CAD build for the part. Positions are in the model's coordinates, mm. Face numbers are marked on the shaded views. A direction names the side the tool comes from. Round coordinates to 2 decimals unless told otherwise and drop trailing zeros. Loops run counter-clockwise (first coordinate to the right, second up) from the corner with the lowest first, then second, coordinate; pieces in that order, holes last. Notation, with made-up numbers: M 60,-20.75 L 92,-20.75 A16 ccw 92,-11.75 Z; hole C 52,-20.5 d5. An arc over 180 degrees is marked long. One line per item, written item: value. Start each with the question number.
from build123d import *

# Parameters (mm, degrees)
SKETCH1_W                      = 59.28
SKETCH1_H                      = 38.1
BOSS_EXTRUDE2_DEPTH            = 29.26
SKETCH2_W                      = 15
SKETCH2_H                      = 38.1
BOSS_EXTRUDE3_DEPTH            = 4
SKETCH4_W                      = 44.28
SKETCH4_H                      = 25.7
CUT_EXTRUDE7_DEPTH             = 27.26
SKETCH7_R                      = 4.75
SKETCH8_R                      = 4.807692308
BOSS_EXTRUDE4_DEPTH            = 2
BOSS_EXTRUDE5_DEPTH            = 2
SKETCH15_W                     = 44.28
SKETCH15_H                     = 2
CUT_EXTRUDE9_DEPTH             = 2
BOSS_EXTRUDE6_DEPTH            = 1
F_2_0MM_DOWEL_HOLE1_AT_2_COUNT = 2
F_2_0MM_DOWEL_HOLE1_AT_2_PITCH = 20.32
LPATTERN1_COUNT                = 2
LPATTERN1_PITCH                = 33.15
SKETCH20_W                     = 25.7
SKETCH20_H                     = 27.26
SKETCH20_W_2                   = 14
SKETCH20_H_2                   = 14
CUT_EXTRUDE10_DEPTH            = 11


with BuildPart() as part:
    # Sketch1 → Boss-Extrude2 (new body)
    with BuildSketch(Plane(origin=(0, 0, 0), x_dir=(1, 0, 0), z_dir=(0, 1, 0))):
        with Locations((29.64, 19.05)):
            Rectangle(SKETCH1_W, SKETCH1_H)
    extrude(amount=BOSS_EXTRUDE2_DEPTH)

    # Sketch2 → Boss-Extrude3 (add)
    with BuildSketch(Plane(origin=(0, 29.26, 0), x_dir=(1, 0, 0), z_dir=(0, 1, 0))):
        with Locations((51.78, 19.05)):
            Rectangle(SKETCH2_W, SKETCH2_H)
    extrude(amount=BOSS_EXTRUDE3_DEPTH)

    # Sketch4 → Cut-Extrude7 (cut)
    with BuildSketch(Plane(origin=(0, 29.26, 0), x_dir=(1, 0, 0), z_dir=(0, 1, 0))):
        with Locations((22.14, 19.05)):
            Rectangle(SKETCH4_W, SKETCH4_H)
    extrude(amount=-CUT_EXTRUDE7_DEPTH, mode=Mode.SUBTRACT)

    # Sketch7 → Cut-Loft2 section 0
    with BuildSketch(Plane(origin=(59.28, 0, 0), x_dir=(0, 0, -1), z_dir=(1, 0, 0))):
        with Locations((19.05, 16.63)):
            Circle(SKETCH7_R)
    # Sketch8 → Cut-Loft2 section 1
    with BuildSketch(Plane.ZY.offset(-44.28)):
        with Locations((-19.05, 16.556791368)):
            Circle(SKETCH8_R)
    loft(mode=Mode.SUBTRACT)

    # Sketch13 → Boss-Extrude4 (add)
    with BuildSketch(Plane.XY):
        Polygon((0, 29.26), (0, 0), (59.28, 0), (59.28, 29.26), (59.28, 33.26), (0, 33.26), align=None)
    extrude(amount=BOSS_EXTRUDE4_DEPTH)

    # Sketch14 → Boss-Extrude5 (add)
    with BuildSketch(Plane(origin=(0, 0, -38.1), x_dir=(-1, 0, 0), z_dir=(0, 0, -1))):
        Polygon((-59.28, 0), (0, 0), (0, 29.26), (0, 33.26), (-59.28, 33.26), (-59.28, 29.26), align=None)
    extrude(amount=BOSS_EXTRUDE5_DEPTH)

    # Sketch15 → Cut-Extrude9 (cut)
    with BuildSketch(Plane(origin=(0, 33.26, 0), x_dir=(1, 0, 0), z_dir=(0, 1, 0))):
        with Locations((22.14, -1)):
            Rectangle(SKETCH15_W, SKETCH15_H)
        with Locations((22.14, 39.1)):
            Rectangle(SKETCH15_W, SKETCH15_H)
    extrude(amount=-CUT_EXTRUDE9_DEPTH, mode=Mode.SUBTRACT)

    # Sketch16 → Boss-Extrude6 (add)
    with BuildSketch(Plane.ZY):
        Polygon((-40.1, 31.26), (-38.1, 31.26), (-38.1, 29.26), (-31.9, 29.26), (-31.9, 2), (-6.2, 2), (-6.2, 29.26), (0, 29.26), (0, 31.26), (2, 31.26), (2, 0), (-40.1, 0), align=None)
    extrude(amount=BOSS_EXTRUDE6_DEPTH)

    # Sketch18 → Ø2.0mm Dowel Hole1 (revolve, cut)
    with BuildSketch(Plane(origin=(2.54, 29.26, -2.475), x_dir=(0, 0, 1), z_dir=(1, 0, 0))):
        Polygon((0, 0), (0, 20.600860619), (1, 20), (1, 0), align=None)
    f_2_0mm_dowel_hole1 = revolve(axis=Axis((2.54, 35.61, -2.475), (0, -1, 0)), mode=Mode.SUBTRACT)

    # Ø2.0mm Dowel Hole1 at 2: Ø2.0mm Dowel Hole1 ×2
    with Locations(*[(i * F_2_0MM_DOWEL_HOLE1_AT_2_PITCH, 0, 0) for i in range(1, F_2_0MM_DOWEL_HOLE1_AT_2_COUNT)]):
        add(f_2_0mm_dowel_hole1, mode=Mode.SUBTRACT)

    # LPattern1: Ø2.0mm Dowel Hole1 ×2
    with Locations(*[(0, 0, -i * LPATTERN1_PITCH) for i in range(1, LPATTERN1_COUNT)]):
        add(f_2_0mm_dowel_hole1, mode=Mode.SUBTRACT)

    # LPattern1 copy 1 sketch → LPattern1 copy 1 (revolve, cut)
    with BuildSketch(Plane(origin=(22.86, 29.26, -35.625), x_dir=(0, 0, 1), z_dir=(1, 0, 0))):
        Polygon((0, 0), (0, 20.600860619), (1, 20), (1, 0), align=None)
    revolve(axis=Axis((22.86, 35.61, -35.625), (0, -1, 0)), mode=Mode.SUBTRACT)

    # Sketch20 → Cut-Extrude10 (cut)
    with BuildSketch(Plane.ZY.offset(-44.28)):
        with Locations((-19.05, 15.63)):
            Rectangle(SKETCH20_W, SKETCH20_H)
        with Locations((-19.05, 16.716836028)):
            Rectangle(SKETCH20_W_2, SKETCH20_H_2, mode=Mode.SUBTRACT)
    extrude(amount=-CUT_EXTRUDE10_DEPTH, mode=Mode.SUBTRACT)


solid = part.part
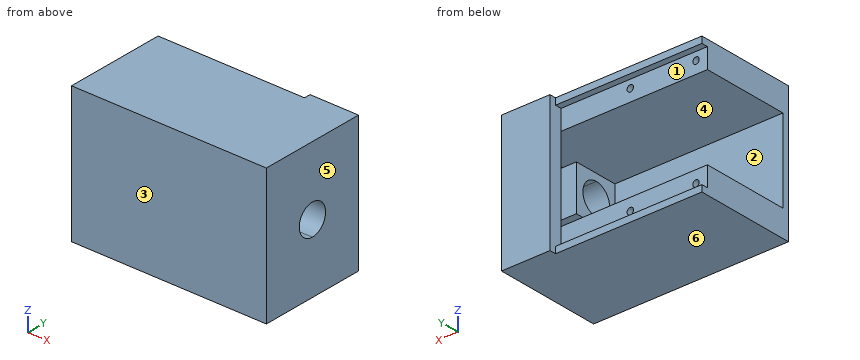
(1) Slice it at A-A, the plane y = 26.5. List the corners of the cut face in (x, z) (3 decimals), and give its area (3 significant figures).
(2) Flat gauge pins, fed straight in: P1, Ø2, axis at y = 31, z = -28.5, coming from the -X side; P2, Ø2.5, axis at x = 22.86, z = -35.625, coming from the -Y side; P3, Ø7, axis at x = 31, z = -33.5, coming from the +Y side; P4, Ø1.6, axis at x = 19, z = -39, coming from the +Y side. Where does each tip first touch, or does it go through?
(3) Slice it at D-D, the plane y = 23. List the corners of the cut face in (x, z) (3 decimals), and give its area (3 significant figures).
(4) Mould opens along Z. For the marked faces 4, 5 and 6 say: pulls with the +Z half, pulls with the -Z half, needs draft (parallel to the pull), parting line crosses it, or undercut.
(5) Probe L1, parallel to Z at x = 22.86, y = 22 (3 decimals); L2, parallel to X at y = 21, z = -2.5; L3, parallel to Z at x = 25, y = 13.5. List the from-to ranges inside material, lowest first.
(6) Which spindle directions (+Z, -Z, +X, -X, +Y, -Y) get a long thin tool onto all of the face, cutting with end or side? Do the marked faces 1, 2 and 3. Say none if no direction does.
(7) Slice it at C-C, the plane x = 30.5. List the corners of the cut face in (y, z), and give its area (3 significant figures).
(8) Slice it at B-B, the plane y = 3. List the corners of the cut face in (x, z).
Check result:
1. outline: M -1,-40.1 L 59.28,-40.1 L 59.28,2 L -1,2 L -1,-6.2 L 55.28,-6.2 L 55.28,-31.9 L -1,-31.9 Z; hole C 2.54,-35.625 d2; hole C 2.54,-2.475 d2; hole C 22.86,-35.625 d2; hole C 22.86,-2.475 d2
1. area: 1,080 mm^2
2. P1: stops at x = 44.28
2. P2: stops at y = 0
2. P3: stops at y = 29.26
2. P4: stops at y = 31.26
3. outline: M -1,-40.1 L 59.28,-40.1 L 59.28,2 L -1,2 L -1,-6.2 L 55.28,-6.2 L 55.28,-12.05 L 44.28,-12.05 L 44.28,-26.05 L 55.28,-26.05 L 55.28,-31.9 L -1,-31.9 Z; hole C 2.54,-35.625 d2; hole C 2.54,-2.475 d2; hole C 22.86,-35.625 d2; hole C 22.86,-2.475 d2
3. area: 1,230 mm^2
4. face 4: undercut
4. face 5: needs draft
4. face 6: pulls with the -Z half
5. L1: z = -40.1 to -36.625, -34.625 to -31.9, -6.2 to -3.475, -1.475 to 2
5. L2: x = -1 to 1.54, 3.54 to 21.86, 23.86 to 59.28
5. L3: z = -40.1 to -31.9, -6.2 to 2
6. face 1: -X, +Y
6. face 2: -X
6. face 3: +Z, -Z, +X, -X, -Y
7. outline: M 0,-40.1 L 31.26,-40.1 L 31.26,-38.1 L 29.26,-38.1 L 29.26,-31.9 L 2,-31.9 L 2,-6.2 L 29.26,-6.2 L 29.26,0 L 31.26,0 L 31.26,2 L 0,2 Z
7. area: 539 mm^2
8. outline: M -1,-40.1 L 59.28,-40.1 L 59.28,2 L -1,2 L -1,-6.2 L 55.28,-6.2 L 55.28,-31.9 L -1,-31.9 Z
